from build123d import *

# Parameters (mm, degrees)
SKETCH5_W           = 145
SKETCH5_H           = 77
BOSS_EXTRUDE2_DEPTH = 17
CHAMFER2_SIZE       = 63
CHAMFER2_SIZE2      = 10
SKETCH1_R           = 2.6
CUT_EXTRUDE1_DEPTH  = 5


with BuildPart() as part:
    # Sketch5 → Boss-Extrude2 (new body)
    with BuildSketch(Plane(origin=(0, 0, 0), x_dir=(1, 0, 0), z_dir=(0, 1, 0))):
        with Locations((72.5, 38.5)):
            Rectangle(SKETCH5_W, SKETCH5_H)
    extrude(amount=BOSS_EXTRUDE2_DEPTH)

    # Chamfer2
    chamfer2_edges = [part.edges().sort_by_distance(p)[0] for p in [
        (72.5, 0, 0),
    ]]
    chamfer2_side = [part.faces().sort_by_distance(p)[0] for p in [
        (72.5, 0, -38.5),
    ]]
    chamfer(chamfer2_edges, length=CHAMFER2_SIZE, length2=CHAMFER2_SIZE2, reference=chamfer2_side[0])

    # Sketch1 → Cut-Extrude1 (cut)
    with BuildSketch(Plane(origin=(0, 17, 0), x_dir=(1, 0, 0), z_dir=(0, 1, 0))):
        with Locations(Location((5, 72, 0), (0, 0, 270))):
            Circle(SKETCH1_R)
        with Locations(Location((5, 5, 0), (0, 0, 270))):
            Circle(SKETCH1_R)
        with Locations(Location((140, 5, 0), (0, 0, 270))):
            Circle(SKETCH1_R)
        with Locations(Location((140, 72, 0), (0, 0, 270))):
            Circle(SKETCH1_R)
    extrude(amount=-CUT_EXTRUDE1_DEPTH, mode=Mode.SUBTRACT)


solid = part.part
Read the model definition and answer for the solid it produces. Units are mm, in the model's axes. A direction names the side the tool comes from. Round coordinates to 2 decimals unless told otherwise and drop trailing zeros. Order: outer loops, then holes, each group sorted by start corner. A loop starts at its lowest first (then second) coordinate and runs counter-clockwise, first axis right, second up.
1) Straight lines are drawn through the part: L1, parallel to X at y = 14.15, z = -5; L2, parallel to Y at x = 89, z = -55; L3, parallel to Y at x = 54.5, z = -13. For each, find the intervals that lie inside material, in ascending order.
2) The part is cut by section B-B on x = 5. Write down the section's boundary in (y, z), plus the area to 3 significant figures.
3) The mould has two halves that part along Z. Classify faces 1 (the face through (140, 12, -5)), 2 (the face through (71.49, 5.07, -31.06)), 3 (the face through (71, 17, -39)), 4 (the face through (137.46, 14.54, -5.56)): released by +Z, released by -Z, zero draft, split by the parting line, or undercut.
4) Flat-ended cylindrical pins translate along their axes: pin 1 (1.5 mm diameter, centred on x = 80, z = -58, fed in from -Y); pin 2 (5.5 mm diameter, centred on x = 140, z = -72, fed in from +Y); pin 3 (5 mm diameter, centred on x = 16, z = -46.5, fed in from -Y); pin 4 (2.5 mm diameter, centred on x = 5, z = -5, fed in from +Y). Find the tip coordinate at first contact, or state that the pin passes through.
5) For faces 5 (the face through (5.78, 14.54, -2.52)), 6 (the face through (0, 10, -47)), determine the directions among +Z, -Z, +X, -X, +Y, -Y from which every point of the face is accessible in a straight line to the end or side of a thin tool.
6) The part is cut by section C-C on y = 7. Write down the section's boundary in (x, z).
7) The part is cut by section D-D on z = -5. Write down the section's boundary in (x, y).
8) The part is cut by section A-A on z = -72. Write down the section's boundary in (x, y), plus the area to 3 significant figures.
Resolved:
1. L1: x = 0 to 2.4, 7.6 to 137.4, 142.6 to 145
1. L2: y = 1.27 to 17
1. L3: y = 7.94 to 17
2. outline: (0, -77) - (17, -77) - (17, -74.6) - (12, -74.6) - (12, -69.4) - (17, -69.4) - (17, -7.6) - (12, -7.6) - (12, -2.4) - (17, -2.4) - (17, 0) - (10, 0) - (0, -63) - close
2. area: 942 mm2
3. face 1: undercut
3. face 2: released by +Z
3. face 3: zero draft
3. face 4: undercut
4. pin 1: stops at y = 0.67
4. pin 2: stops at y = 17
4. pin 3: stops at y = 2.22
4. pin 4: stops at y = 12
5. face 5: +Y
5. face 6: +Z, -Z, -X, +Y, -Y
6. outline: (0, -77) - (145, -77) - (145, -18.9) - (0, -18.9) - close
7. outline: (0, 9.21) - (145, 9.21) - (145, 17) - (142.6, 17) - (142.6, 12) - (137.4, 12) - (137.4, 17) - (7.6, 17) - (7.6, 12) - (2.4, 12) - (2.4, 17) - (0, 17) - close
8. outline: (0, 0) - (145, 0) - (145, 17) - (142.6, 17) - (142.6, 12) - (137.4, 12) - (137.4, 17) - (7.6, 17) - (7.6, 12) - (2.4, 12) - (2.4, 17) - (0, 17) - close
8. area: 2,410 mm2
